from build123d import *

# Parameters (mm, degrees)
F0_R     = 7.5
F1_DEPTH = 2
F3_DEPTH = 2


with BuildPart() as f1:
    # F0 (on Top) → F1 (new body)
    with BuildSketch(Plane.XY):
        Circle(F0_R)
    extrude(amount=F1_DEPTH)

    # F2 (on face) → F3 (join)
    with BuildSketch(Plane.XY.offset(2)):
        with BuildLine():
            Line((-0.35, 5.853991), (-2.454586, 5.853991))
            Line((-2.454586, 5.853991), (-2.454586, 5.153991))
            Line((-2.454586, 5.153991), (-0.35, 5.153991))
            Line((-0.35, 5.153991), (-0.35, 4.102806))
            ThreePointArc((-0.35, 4.102806), (-2.911659, 2.911659), (-4.102806, 0.35))
            Line((-4.102806, 0.35), (-5.201799, 0.35))
            Line((-5.201799, 0.35), (-5.201799, 2.505629))
            Line((-5.201799, 2.505629), (-5.901799, 2.505629))
            Line((-5.901799, 2.505629), (-5.901799, 0))
            Line((-5.901799, 0), (-5.901799, -2.505629))
            Line((-5.901799, -2.505629), (-5.201799, -2.505629))
            Line((-5.201799, -2.505629), (-5.201799, -0.35))
            Line((-5.201799, -0.35), (-4.102806, -0.35))
            ThreePointArc((-4.102806, -0.35), (-2.911659, -2.911659), (-0.35, -4.102806))
            Line((-0.35, -4.102806), (-0.35, -5.153991))
            Line((-0.35, -5.153991), (-2.454586, -5.153991))
            Line((-2.454586, -5.153991), (-2.454586, -5.853991))
            Line((-2.454586, -5.853991), (0, -5.853991))
            Line((0, -5.853991), (2.454586, -5.853991))
            Line((2.454586, -5.853991), (2.454586, -5.153991))
            Line((2.454586, -5.153991), (0.35, -5.153991))
            Line((0.35, -5.153991), (0.35, -4.102806))
            ThreePointArc((0.35, -4.102806), (2.911659, -2.911659), (4.102806, -0.35))
            Line((4.102806, -0.35), (5.201799, -0.35))
            Line((5.201799, -0.35), (5.201799, -2.505629))
            Line((5.201799, -2.505629), (5.901799, -2.505629))
            Line((5.901799, -2.505629), (5.901799, 0))
            Line((5.901799, 0), (5.901799, 2.505629))
            Line((5.901799, 2.505629), (5.201799, 2.505629))
            Line((5.201799, 2.505629), (5.201799, 0.35))
            Line((5.201799, 0.35), (4.102806, 0.35))
            ThreePointArc((4.102806, 0.35), (2.911659, 2.911659), (0.35, 4.102806))
            Line((0.35, 4.102806), (0.35, 5.153991))
            Line((0.35, 5.153991), (2.454586, 5.153991))
            Line((2.454586, 5.153991), (2.454586, 5.853991))
            Line((2.454586, 5.853991), (0, 5.853991))
            Line((0, 5.853991), (-0.35, 5.853991))
        make_face()
        with BuildLine():
            Line((-3.70601, -0.35), (-0.35, -0.35))
            Line((-0.35, -0.35), (-0.35, -3.70601))
            ThreePointArc((-0.35, -3.70601), (-2.632205, -2.632205), (-3.70601, -0.35))
        make_face(mode=Mode.SUBTRACT)
        with BuildLine():
            Line((0.35, -3.70601), (0.35, -0.35))
            Line((0.35, -0.35), (3.70601, -0.35))
            ThreePointArc((3.70601, -0.35), (2.632205, -2.632205), (0.35, -3.70601))
        make_face(mode=Mode.SUBTRACT)
        with BuildLine():
            Line((-0.35, 3.70601), (-0.35, 0.35))
            Line((-0.35, 0.35), (-3.70601, 0.35))
            ThreePointArc((-3.70601, 0.35), (-2.632205, 2.632205), (-0.35, 3.70601))
        make_face(mode=Mode.SUBTRACT)
        with BuildLine():
            Line((3.70601, 0.35), (0.35, 0.35))
            Line((0.35, 0.35), (0.35, 3.70601))
            ThreePointArc((0.35, 3.70601), (2.632205, 2.632205), (3.70601, 0.35))
        make_face(mode=Mode.SUBTRACT)
    extrude(amount=F3_DEPTH)


solid = f1.part
Design review of the part built by this model. Coordinates are the model's own, in mm. A direction names the side the tool comes from. Coordinates: 2 decimals unless noted, no trailing zeros. Loops run counter-clockwise (first coordinate to the right, second up) from the corner with the lowest first, then second, coordinate; pieces in that order, holes last. Notation, with made-up numbers: (44.5, -24.75) -> (98.5, -24.75) arc R20 ccw to (98.5, -6.75) -> close; hole circle Ø3 at (-23.75, 43). An arc over 180 degrees is marked (long way). Use a Markdown table: item, result. Add a question column.
Item 1: The part is to be moulded in two halves that separate along X. For faces 5 (the flat face through (-1, -5.154, 3)), 6 (the cylindrical face through (-2.607, -2.658, 2.986)), 7 (the flat face through (-5.902, 0, 3)), say which applies: +X half, -X half, draft (parallel to the pull), parting line (faces both ways), or undercut.
Item 2: We need section C-C, the plane z = 2.7. Count the separate pieces of the cut face and the enclosed holes in it, and give its area (3 significant figures).
Item 3: We need section B-B, the plane x = 0. Write out the cut boundary in (y, z).
Item 4: We need section A-A, the plane y = 0. Write out the cut boundary in (x, z), and give its area (3 significant figures).
Item 5: Machinability: for faces 1 (the flat face through (-5.202, -1, 3)), 2 (the cylindrical face through (2.94, 2.883, 2.986)), 3 (the flat face through (0.35, 5, 3)), 4 (the flat face through (-5.202, 1, 3)), which of the approach directions +Z, -Z, +X, -X, +Y, -Y give a long, thin tool a straight path to every point of the face, cutting with its end or side? Answer none if there is none.
Item 6: Wall thickness on L1, parallel to X at y = -2, z = 3.1; L2, parallel to Y at x = -3, z = 2.8; L3, parallel to Y at x = 2.25, z = 3.1: over which ranges is each line inside the solid? List them lowest first. Write a range as from..to.
Item 7: We need section D-D, the plane x = 3. Write out the cut boundary in (y, z), and give its area (3 significant figures).
Item 8: Clearance check with flat-ended pins moving along their axes: P1, Ø2, axis at y = 2, z = 3.5, coming from the -X side; P2, Ø0.6, axis at x = 2, z = 2.5, coming from the +Y side; P3, Ø2, axis at x = 3.5, z = 0.5, coming from the +Y side. State where each tip first meets the part, or that it passes through.
Numbers:
| question | item | result |
|---|---|---|
| 1 | face 5 | draft |
| 1 | face 6 | undercut |
| 1 | face 7 | -X half |
| 2 | separate pieces | 1 |
| 2 | enclosed holes | 4 |
| 2 | area | 36.5 mm^2 |
| 3 | outline | (-7.5, 0) -> (7.5, 0) -> (7.5, 2) -> (5.85, 2) -> (5.85, 4) -> (-5.85, 4) -> (-5.85, 2) -> (-7.5, 2) -> close |
| 4 | outline | (-7.5, 0) -> (7.5, 0) -> (7.5, 2) -> (5.9, 2) -> (5.9, 4) -> (-5.9, 4) -> (-5.9, 2) -> (-7.5, 2) -> close |
| 4 | area | 53.6 mm^2 |
| 5 | face 1 | +Z, -Y |
| 5 | face 2 | +Z |
| 5 | face 3 | +Z, +X |
| 5 | face 4 | +Z, +Y |
| 6 | L1 | x = -5.9..-5.2, -3.6..-3.14, -0.35..0.35, 3.14..3.6, 5.2..5.9 |
| 6 | L2 | y = -2.82..-2.2, -0.35..0.35, 2.2..2.82 |
| 6 | L3 | y = -5.85..-5.15, -3.45..-2.97, -0.35..0.35, 2.97..3.45, 5.15..5.85 |
| 7 | outline | (-6.87, 0) -> (6.87, 0) -> (6.87, 2) -> (2.82, 2) -> (2.82, 4) -> (2.2, 4) -> (2.2, 2) -> (0.35, 2) -> (0.35, 4) -> (-0.35, 4) -> (-0.35, 2) -> (-2.2, 2) -> (-2.2, 4) -> (-2.82, 4) -> (-2.82, 2) -> (-6.87, 2) -> close |
| 7 | area | 31.4 mm^2 |
| 8 | P1 | stops at x = -5.9 |
| 8 | P2 | stops at y = 5.85 |
| 8 | P3 | stops at y = 7.07 |
